```python
from build123d import *

# Parameters (mm, degrees)
SKETCH1_R           = 10
SKETCH1_R_2         = 5
BOSS_EXTRUDE1_DEPTH = 10
SKETCH2_R           = 12.5
BOSS_EXTRUDE2_DEPTH = 10
SKETCH3_R           = 5
CUT_EXTRUDE1_DEPTH  = 10
CUT_EXTRUDE4_DEPTH  = 10


with BuildPart() as part:
    # Sketch1 → Boss-Extrude1 (new body)
    with BuildSketch(Plane.XY):
        Circle(SKETCH1_R)
        Circle(SKETCH1_R_2, mode=Mode.SUBTRACT)
    extrude(amount=BOSS_EXTRUDE1_DEPTH)

    # Sketch2 → Boss-Extrude2 (add)
    with BuildSketch(Plane(origin=(0, 0, 0), x_dir=(-1, 0, 0), z_dir=(0, 0, -1))):
        Circle(SKETCH2_R)
    extrude(amount=-BOSS_EXTRUDE2_DEPTH)

    # Sketch3 → Cut-Extrude1 (cut)
    with BuildSketch(Plane(origin=(0, 0, 0), x_dir=(-1, 0, 0), z_dir=(0, 0, -1))):
        Circle(SKETCH3_R)
    extrude(amount=-CUT_EXTRUDE1_DEPTH, mode=Mode.SUBTRACT)

    # Sketch4 → Cut-Extrude4 (cut)
    with BuildSketch(Plane(origin=(0, 0, 0), x_dir=(-1, 0, 0), z_dir=(0, 0, -1))):
        with BuildLine():
            Line((-9.669699641, 8.08598777), (-7.258106214, 6.878945717))
            ThreePointArc((-7.258106214, 6.878945717), (-6.46463523, 7.629448954), (-5.59405076, 8.288944209))
            Line((-5.59405076, 8.288944209), (-6.390582917, 10.864931631))
            ThreePointArc((-6.390582917, 10.864931631), (-8.149466314, 9.616261652), (-9.669699641, 8.08598777))
        make_face()
        with BuildLine():
            Line((-5.544842662, 11.31993857), (-3.832690674, 9.23636737))
            ThreePointArc((-3.832690674, 9.23636737), (-2.802561694, 9.599252468), (-1.73900232, 9.847632758))
            Line((-1.73900232, 9.847632758), (-1.418922177, 12.524893183))
            ThreePointArc((-1.418922177, 12.524893183), (-3.53362195, 12.099578724), (-5.544842662, 11.31993857))
        make_face()
        with BuildLine():
            Line((-0.461232014, 12.596569152), (0.255431902, 9.996737195))
            ThreePointArc((0.255431902, 9.996737195), (1.34410022, 9.909258025), (2.41673542, 9.70357614))
            Line((2.41673542, 9.70357614), (3.798083099, 12.019186917))
            ThreePointArc((3.798083099, 12.019186917), (1.693217751, 12.490768712), (-0.461232014, 12.596569152))
        make_face()
        with BuildLine():
            Line((4.70212984, 11.695138492), (4.299387983, 9.028580341))
            ThreePointArc((4.299387983, 9.028580341), (5.258354995, 8.505862846), (6.15459765, 7.881683054))
            Line((6.15459765, 7.881683054), (8.358365302, 9.435254043))
            ThreePointArc((8.358365302, 9.435254043), (6.627284721, 10.722191316), (4.70212984, 11.695138492))
        make_face()
        with BuildLine():
            Line((9.052450727, 8.771512139), (7.599940822, 6.499299924))
            ThreePointArc((7.599940822, 6.499299924), (8.26339242, 5.631726707), (8.828274034, 4.696975365))
            Line((8.828274034, 4.696975365), (11.473410211, 5.219880028))
            ThreePointArc((11.473410211, 5.219880028), (10.415433955, 7.099649632), (9.052450727, 8.771512139))
        make_face()
        with BuildLine():
            Line((11.837520645, 4.331211651), (9.58639485, 2.846231506))
            ThreePointArc((9.58639485, 2.846231506), (9.839614226, 1.783813859), (9.975461635, 0.700117964))
            Line((9.975461635, 0.700117964), (12.604598262, 0.101941336))
            ThreePointArc((12.604598262, 0.101941336), (12.402660038, 2.249514029), (11.837520645, 4.331211651))
        make_face()
        with BuildLine():
            Line((12.575775702, -0.857994679), (9.915274118, -1.298976196))
            ThreePointArc((9.915274118, -1.298976196), (9.714477342, -2.372536612), (9.397801295, -3.417796193))
            Line((9.397801295, -3.417796193), (11.556336764, -5.03362394))
            ThreePointArc((11.556336764, -5.03362394), (12.245353525, -2.989582985), (12.575775702, -0.857994679))
        make_face()
        with BuildLine():
            Line((11.139564893, -5.898845935), (8.529712414, -5.219579114))
            ThreePointArc((8.529712414, -5.219579114), (7.909619072, -6.118653948), (7.195175735, -6.944742338))
            Line((7.195175735, -6.944742338), (8.509879654, -9.298829908))
            ThreePointArc((8.509879654, -9.298829908), (9.970714142, -7.711753943), (11.139564893, -5.898845935))
        make_face()
        with BuildLine():
            Line((7.777222115, -9.919733139), (5.669285944, -8.237669384))
            ThreePointArc((5.669285944, -8.237669384), (4.737115808, -8.80680043), (3.748438924, -9.270879442))
            Line((3.748438924, -9.270879442), (3.991987042, -11.956183707))
            ThreePointArc((3.991987042, -11.956183707), (5.972047703, -11.100492584), (7.777222115, -9.919733139))
        make_face()
        with BuildLine():
            Line((3.070126979, -12.225408366), (1.82858843, -9.831391781))
            ThreePointArc((1.82858843, -9.831391781), (0.745522186, -9.972171111), (-0.34643703, -9.993997268))
            Line((-0.34643703, -9.993997268), (-1.216156396, -12.546204725))
            ThreePointArc((-1.216156396, -12.546204725), (0.940759962, -12.569855213), (3.070126979, -12.225408366))
        make_face()
        with BuildLine():
            Line((-2.167821003, -12.417199422), (-2.328288635, -9.725177224))
            ThreePointArc((-2.328288635, -9.725177224), (-3.374978996, -9.413262813), (-4.381410875, -8.989062173))
            Line((-4.381410875, -8.989062173), (-6.214015345, -10.966872967))
            ThreePointArc((-6.214015345, -10.966872967), (-4.253193723, -11.865775682), (-2.167821003, -12.417199422))
        make_face()
        with BuildLine():
            Line((-7.03093304, -10.461943891), (-6.082583444, -7.937391174))
            ThreePointArc((-6.082583444, -7.937391174), (-6.911915648, -7.226715857), (-7.658798975, -6.429836565))
            Line((-7.658798975, -6.429836565), (-10.137414587, -7.491269242))
            ThreePointArc((-10.137414587, -7.491269242), (-8.711731575, -9.109995738), (-7.03093304, -10.461943891))
        make_face()
        with BuildLine():
            Line((-10.678332879, -6.697723217), (-8.785144317, -4.777158081))
            ThreePointArc((-8.785144317, -4.777158081), (-9.253719292, -3.790604077), (-9.611911155, -2.758833802))
            Line((-9.611911155, -2.758833802), (-12.307962753, -2.72035701))
            ThreePointArc((-12.307962753, -2.72035701), (-11.663931893, -4.77901477), (-10.678332879, -6.697723217))
        make_face()
        with BuildLine():
            Line((-12.479351955, -1.775405353), (-9.968673927, -0.790910957))
            ThreePointArc((-9.968673927, -0.790910957), (-9.995470803, 0.300937585), (-9.903036574, 1.389196388))
            Line((-9.903036574, 1.389196388), (-12.350352343, 2.520929664))
            ThreePointArc((-12.350352343, 2.520929664), (-12.599332424, 0.378301268), (-12.479351955, -1.775405353))
        make_face()
        with BuildLine():
            Line((-12.122577706, 3.453896227), (-9.428529252, 3.332091857))
            ThreePointArc((-9.428529252, 3.332091857), (-9.008914606, 4.340444404), (-8.481837004, 5.297021903))
            Line((-8.481837004, 5.297021903), (-10.257253815, 7.326324696))
            ThreePointArc((-10.257253815, 7.326324696), (-11.356193917, 5.47020558), (-12.122577706, 3.453896227))
        make_face()
    extrude(amount=-CUT_EXTRUDE4_DEPTH, mode=Mode.SUBTRACT)


solid = part.part
```
Check sheet for the modelled part. Datum: model origin and axes. Units: mm. A direction names the side the tool comes from. Give positions to 0.01 mm unless a question says otherwise; leave off trailing zeros. Order: outer loops, then holes, each group sorted by start corner. A loop starts at its lowest first (then second) coordinate and runs counter-clockwise, first axis right, second up. Notation, with made-up numbers: M 16.25,-37.5 L 54.25,-37.5 A26 ccw 54.25,-23.5 Z; hole C -39.75,14.5 d8. An arc over 180 degrees is marked long. Answer in a Markdown table with one row per item. Add a question column.
Q1. Access from +Z, -Z, +X, -X, +Y, -Y to the whole of each face (thin tool, end or side, straight path). Record for faces 4 (the flat face through (-8.31, 7.61, 4.93)), 5 (the flat face through (8.432, 7.466, 4.93)), 6 (the flat face through (2.25, -11.04, 4.93)).
Q2. Thickness scan on L1, parallel to X at y = 4, z = 4; L2, parallel to Y at x = -1.25, z = 9.25; L3, parallel to X at y = 3.75, z = 7.25. Record the ranges inside material, lowest first.
Q3. Release check for a two-part mould opening along X. For faces 1 (the cylindrical face through (10.333, -7.035, 4.93)), 2 (the cylindrical face through (-9.837, 1.799, 4.93)), 3 (the flat face through (-9.8, -5.55, 4.93)) record: released by +X, released by -X, zero draft, split by the parting line, or undercut.
Q4. Gauge pin test, flat ends, axial feed: pin 1 Ø5 at (y, z) = (-3, 3.5) entering from -X; pin 2 Ø1 at (x, z) = (8.5, 7) entering from +Y; pin 3 Ø10 at (x, y) = (-3, -3.5) entering from -Z; pin 4 Ø5 at (x, z) = (-4.5, 4.5) entering from -Y. Record the tip position at first contact, or that the pin passes through.
Q5. Sectioned sample at A-A, the plane y = 1. Record the boundary of the cut face in (x, z).
Verdict:
| question | item | result |
|---|---|---|
| 1 | face 4 | +Z, -Z, -X |
| 1 | face 5 | +Z, -Z, +Y |
| 1 | face 6 | +Z, -Z, -Y |
| 2 | L1 | -11.34 to -3, 3 to 9.17 |
| 2 | L2 | -9.92 to -4.84, 4.84 to 9.92 |
| 2 | L3 | -10.96 to -3.31, 3.31 to 9.27 |
| 3 | face 1 | released by +X |
| 3 | face 2 | released by -X |
| 3 | face 3 | undercut |
| 4 | pin 1 | x = -12.49 |
| 4 | pin 2 | y = 7.75 |
| 4 | pin 3 | z = 0 |
| 4 | pin 4 | y = -12.13 |
| 5 | outline | M -9.95,0 L -4.9,0 L -4.9,10 L -9.95,10 Z; M 4.9,0 L 9.95,0 L 9.95,10 L 4.9,10 Z |
